```python
from build123d import *

# Parameters (mm, degrees)
SKETCH1_W                  = 100
SKETCH1_H                  = 100
MAINBODY_DEPTH             = 5
SKETCH2_R                  = 6.5
SKETCH2_R_2                = 4
BEARING_BUSHINGHOLES_DEPTH = 6
M4_TAPPED_HOLE1_D          = 3.3
SKETCH5_R                  = 1.65
SKETCH5_R_2                = 4
CUT_EXTRUDE1_DEPTH         = 6


with BuildPart() as part:
    # Sketch1 → MainBody (new body)
    with BuildSketch(Plane.XY):
        Rectangle(SKETCH1_W, SKETCH1_H)
    extrude(amount=MAINBODY_DEPTH)

    # Sketch2 → Bearing&BushingHoles (cut, through all)
    with BuildSketch(Plane.XY.offset(5)):
        Circle(SKETCH2_R)
        with Locations((-42.928932188, -42.928932188)):
            Circle(SKETCH2_R_2)
        with Locations((42.928932188, -42.928932188)):
            Circle(SKETCH2_R_2)
        with Locations((42.928932188, 42.928932188)):
            Circle(SKETCH2_R_2)
        with Locations((-42.928932188, 42.928932188)):
            Circle(SKETCH2_R_2)
    extrude(amount=-BEARING_BUSHINGHOLES_DEPTH, mode=Mode.SUBTRACT)

    # M4 Tapped Hole1 (through all)
    with Locations(Plane(origin=(-39.597979746, -28.991378029, 0), x_dir=(-1, 0, 0), z_dir=(0, 0, -1))):
        with Locations((0, 0), (-10.606601717, -10.606601717), (-68.589357775, 68.589357775), (-79.195959492, 57.982756058)):
            Hole(M4_TAPPED_HOLE1_D / 2)

    # Sketch5 → Cut-Extrude1 (cut, through all)
    with BuildSketch(Plane(origin=(0, 0, 0), x_dir=(-1, 0, 0), z_dir=(0, 0, -1))):
        with Locations((28.991378029, -39.597979746)):
            Circle(SKETCH5_R)
        with Locations((39.597979746, -28.991378029)):
            Circle(SKETCH5_R)
        with Locations((42.928932188, 42.928932188)):
            Circle(SKETCH5_R_2)
        with Locations((-39.597979746, 28.991378029)):
            Circle(SKETCH5_R)
        with Locations((-28.991378029, 39.597979746)):
            Circle(SKETCH5_R)
        with BuildLine():
            Line((-44, 27.493139834), (-44, -36.011359367))
            ThreePointArc((-44, -36.011359367), (-42.268855308, -35.960123214), (-40.578116577, -36.33547589))
            Line((-40.578116577, -36.33547589), (-10.701821494, -6.459180807))
            ThreePointArc((-10.701821494, -6.459180807), (-12.5, 0), (-10.701821494, 6.459180807))
            Line((-10.701821494, 6.459180807), (-35.587597155, 31.344956468))
            ThreePointArc((-35.587597155, 31.344956468), (-37.66214198, 24.763490596), (-44, 27.493139834))
        make_face()
        with BuildLine():
            Line((44, -27.493139834), (44, 36.011359367))
            ThreePointArc((44, 36.011359367), (42.268855308, 35.960123214), (40.578116577, 36.33547589))
            Line((40.578116577, 36.33547589), (10.701821494, 6.459180807))
            ThreePointArc((10.701821494, 6.459180807), (12.5, 0), (10.701821494, -6.459180807))
            Line((10.701821494, -6.459180807), (35.587597155, -31.344956468))
            ThreePointArc((35.587597155, -31.344956468), (37.66214198, -24.763490596), (44, -27.493139834))
        make_face()
        with BuildLine():
            Line((-27.493139834, 44), (36.011359367, 44))
            ThreePointArc((36.011359367, 44), (35.960123214, 42.268855308), (36.33547589, 40.578116577))
            Line((36.33547589, 40.578116577), (6.459180807, 10.701821494))
            ThreePointArc((6.459180807, 10.701821494), (0, 12.5), (-6.459180807, 10.701821494))
            Line((-6.459180807, 10.701821494), (-31.344956468, 35.587597155))
            ThreePointArc((-31.344956468, 35.587597155), (-24.763490596, 37.66214198), (-27.493139834, 44))
        make_face()
        with BuildLine():
            Line((6.459180807, -10.701821494), (31.344956468, -35.587597155))
            ThreePointArc((31.344956468, -35.587597155), (24.763490596, -37.66214198), (27.493139834, -44))
            Line((27.493139834, -44), (-36.011359367, -44))
            ThreePointArc((-36.011359367, -44), (-35.960123214, -42.268855308), (-36.33547589, -40.578116577))
            Line((-36.33547589, -40.578116577), (-6.459180807, -10.701821494))
            ThreePointArc((-6.459180807, -10.701821494), (0, -12.5), (6.459180807, -10.701821494))
        make_face()
    extrude(amount=-CUT_EXTRUDE1_DEPTH, mode=Mode.SUBTRACT)


solid = part.part
```
Read the model definition and answer for the solid it produces. Units are mm, in the model's axes. A direction names the side the tool comes from. Coordinates: 2 decimals unless noted, no trailing zeros. Loops run counter-clockwise (first coordinate to the right, second up) from the corner with the lowest first, then second, coordinate; pieces in that order, holes last.
(1) The mould has two halves that part along Y. Classify faces 3 (the face through (42.29, -35.96, 2.46)), 4 (the face through (44, -4, 2)), 5 (the face through (-1, -50, 2)), 6 (the face through (-50, -1, 2)): released by +Y, released by -Y, zero draft, split by the parting line, or undercut.
Solution:
face 3: undercut
face 4: undercut
face 5: released by -Y
face 6: zero draft
(2) The part is cut by section C-C (z = 4). Count the separate pieces of the cut face and the enclosed holes in it, and give its area (3 significant figures).
Solution:
separate pieces: 1
enclosed holes: 13
area: 3,930 mm2
(3) A tool of negligible diameter and unlimited length cuts with its end or side. For faces 1 (the face through (-4, 44, 2)), 2 (the face through (-12, 12, 0)), from which of +Z, -Z, +X, -X, +Y, -Y can it reach the whole face along a straight path? Write none if from no direction.
Solution:
face 1: +Z, -Z
face 2: -Z, +X, -X, +Y, -Y
(4) Consider line 1 along X through (y, z) = (-41, 1.35); line 2 along X through (y, z) = (21, 0.5); line 3 along X through (y, z) = (7, 1.5). Determine where each line is inside the solid, lowest interval first.
Solution:
line 1: x = -50 to -46.43, -39.42 to -29.86, -28.12 to -24.56, 36.2 to 39.42, 46.43 to 50
line 2: x = -50 to -44, -25.24 to -16.76, 16.76 to 25.24, 44 to 50
line 3: x = -50 to -44, -11.24 to 11.24, 44 to 50
(5) The part is cut by section A-A (y = 0). Determine the outline of the cut face in (x, z).
Solution:
outline: (-50, 0) - (-44, 0) - (-44, 5) - (-50, 5) - close; (-12.5, 0) - (-6.5, 0) - (-6.5, 5) - (-12.5, 5) - close; (6.5, 0) - (12.5, 0) - (12.5, 5) - (6.5, 5) - close; (44, 0) - (50, 0) - (50, 5) - (44, 5) - close
(6) A flat-ended cylindrical pin translates along its axis: pin 1 Ø7 at (x, y) = (42.93, -42.93) entering from +Z. Find the tip coordinate at first contact, or state that the pin passes through.
Solution:
pin 1: passes through
